Here's how the part is built. I have some questions about the finished solid (model axes, mm). Give positions to 0.01 mm unless a question says otherwise; leave off trailing zeros. Loops run counter-clockwise (first coordinate to the right, second up) from the corner with the lowest first, then second, coordinate; pieces in that order, holes last. Notation, with made-up numbers: (54.5, -26) -> (84.5, -26) arc R27 ccw to (84.5, -6) -> close; hole circle Ø1 at (58, 42). An arc over 180 degrees is marked (long way). Answer in a Markdown table with one row per item. Add a question column.
Item 1: If we section it at D-D (z = -180.5): Write out the boundary of the cut face in (x, y).
Item 2: If we section it at B-B (x = -67): Write out the boundary of the cut face in (y, z).
Item 3: If I drill on line 1 (Z direction, x = -72.5, y = 1.25); line 2 (X direction, y = 1.5, z = -121); line 3 (X direction, y = 6.25, z = -209), over which ranges is the centre line in solid material (lowest first)?
Item 4: If we section it at A-A (z = -123.5): Write out the boundary of the cut face in (x, y).
```python
from build123d import *

# Parameters (mm, degrees)
BOSS_EXTRUDE1_DEPTH = 6.35
SKETCH3_W           = 19.05
SKETCH3_H           = 169.388632852
CUT_EXTRUDE3_DEPTH  = 327.660693329
CUT_EXTRUDE2_DEPTH  = 327.660693329


with BuildPart() as part:
    # Sketch1 → Boss-Extrude1 (new body)
    with BuildSketch(Plane(origin=(0, 0, 0), x_dir=(1, 0, 0), z_dir=(0, 1, 0))):
        with BuildLine():
            Line((0, 169.388632852), (0, 0))
            Line((0, 0), (-19.05, 0))
            ThreePointArc((-19.05, 0), (-39.88804557, 37.868270719), (-73.722410895, 64.765590165))
            ThreePointArc((-73.722410895, 64.765590165), (-54.193392954, 116.375662835), (-38.876501861, 169.388632852))
            ThreePointArc((-38.876501861, 169.388632852), (-39.194658591, 248.155900408), (-76.554791267, 317.5))
            Line((-76.554791267, 317.5), (-19.05, 317.5))
            Line((-19.05, 317.5), (-19.05, 169.388632852))
            Line((-19.05, 169.388632852), (0, 169.388632852))
        make_face()
    extrude(amount=BOSS_EXTRUDE1_DEPTH)

    # Sketch3 → Cut-Extrude3 (cut, through all)
    with BuildSketch(Plane(origin=(0, 6.35, 0), x_dir=(1, 0, 0), z_dir=(0, 1, 0))):
        with Locations((-9.525, 84.694316426)):
            Rectangle(SKETCH3_W, SKETCH3_H)
    extrude(amount=-CUT_EXTRUDE3_DEPTH, mode=Mode.SUBTRACT)

    # Sketch2 → Cut-Extrude2 (cut, through all)
    with BuildSketch(Plane(origin=(0, 6.35, 0), x_dir=(1, 0, 0), z_dir=(0, 1, 0))):
        Polygon((-39.164098049, 109.561842364), (-23.543572116, 153.825683885), (-32.944847981, 157.143355113), (-37.133143759, 145.274992843), (-40.27089443, 146.38229203), (-43.588565658, 136.981016166), (-39.696317688, 135.607458014), (-47.810876614, 112.613254626), align=None)
    extrude(amount=-CUT_EXTRUDE2_DEPTH, mode=Mode.SUBTRACT)


solid = part.part
```
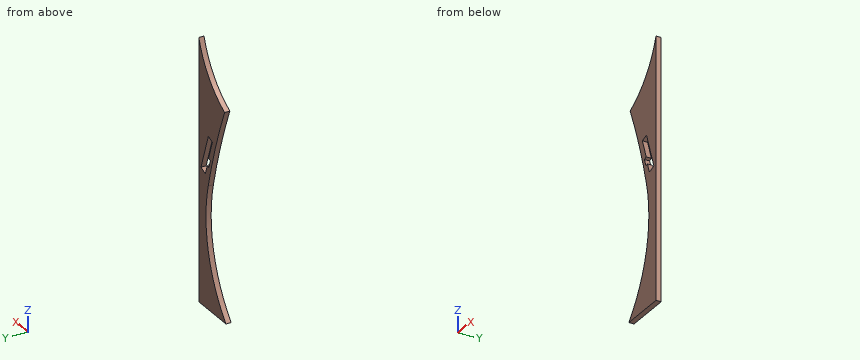
Recorded:
| question | item | result |
|---|---|---|
| 1 | outline | (-36.55, 0) -> (-19.05, 0) -> (-19.05, 6.35) -> (-36.55, 6.35) -> close |
| 2 | outline | (0, -317.5) -> (6.35, -317.5) -> (6.35, -306) -> (0, -306) -> close; (0, -81.16) -> (6.35, -81.16) -> (6.35, -61.02) -> (0, -61.02) -> close |
| 3 | line 1 | z = -317.5 to -312.88, -67.66 to -64.13 |
| 3 | line 2 | x = -52.67 to -44.85, -35.13 to -19.05 |
| 3 | line 3 | x = -34.19 to -19.05 |
| 4 | outline | (-51.86, 0) -> (-43.97, 0) -> (-43.97, 6.35) -> (-51.86, 6.35) -> close; (-34.25, 0) -> (-19.05, 0) -> (-19.05, 6.35) -> (-34.25, 6.35) -> close |
